Source: CAD feature listing. Evaluate the final solid. Frame: model axes, mm. Face numbers are marked on the shaded views. A direction names the side the tool comes from. Round coordinates to 2 decimals unless told otherwise and drop trailing zeros. Order: outer loops, then holes, each group sorted by start corner. A loop starts at its lowest first (then second) coordinate and runs counter-clockwise, first axis right, second up. Notation, with made-up numbers: (17.25, 18.25) -> (24.25, 18.25) arc R24 ccw to (24.25, 53.25) -> close; hole circle Ø11 at (64.5, -19). An arc over 180 degrees is marked (long way). Use a Markdown table: item, result. Add a question column.
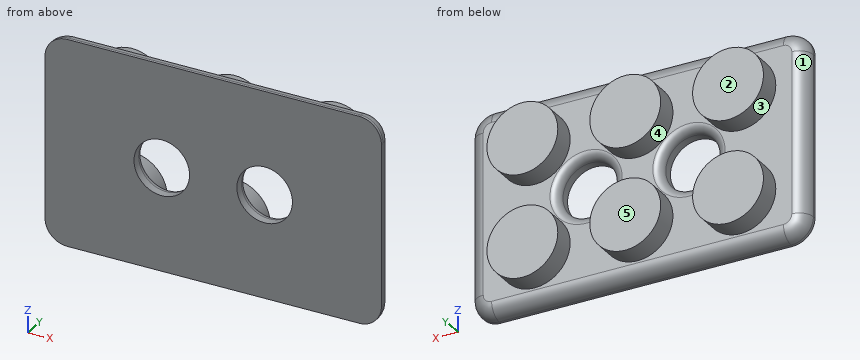
Autodesk Inventor part; units mm, degrees
ref_plane "YZ Plane" through (0, 0, 0) normal (1, 0, 0) x (0, 1, 0)
ref_plane "XZ Plane" through (0, 0, 0) normal (0, 1, 0) x (-1, 0, 0)
ref_plane "XY Plane" through (0, 0, 0) normal (0, 0, 1) x (1, 0, 0)
sketch "Sketch1" plane through (0, 0, 0) normal (0, 1, 0) x (-1, 0, 0)
  line L0 (25.9, 0) -> (-25.9, 0)
  line L1 (0, -25.9) -> (0, 25.9)
  circle A0 centre (0, 0) radius 18.5 construction
  circle A1 centre (0, 0) radius 13 construction
  dimension "d0" = 37
  dimension "d1" = 26
sketch "Sketch2" plane through (0, 0, 0) normal (0, 1, 0) x (-1, 0, 0)
  line L0 (84.7, 0) -> (-84.7, 0)
  line L1 (0, -33.3) -> (0, 70.3)
  line L2 (-60.5, 55.5) -> (-60.5, -18.5)
  line L3 (-60.5, -18.5) -> (60.5, -18.5)
  line L4 (60.5, -18.5) -> (60.5, 55.5)
  line L5 (-60.5, 55.5) -> (60.5, 55.5)
  circle A0 centre (0, 37) radius 18.5 construction
  point P0 (0, 0)
  dimension "d3" = 121
  dimension "d29" = 18.5
  dimension "d30" = 55.5
  dimension "d99" = 37
  dimension "d100" = 37
extrude "Extrusion1" add sketch "Sketch2" along normal blind 6
sketch "Sketch6" plane through (0, 0, 0) normal (0, 1, 0) x (-1, 0, 0)
  line L0 (60.5, -18.5) -> (-60.5, -18.5)
  line L1 (60.5, 55.5) -> (60.5, -18.5)
  line L2 (-60.5, -18.5) -> (60.5, -18.5)
  line L3 (60.5, -18.5) -> (60.5, 55.5)
  line L4 (-60.5, 55.5) -> (-60.5, -18.5)
  line L5 (84.7, 0) -> (-84.7, 0)
  line L6 (0, -36.3) -> (0, 70.8)
  arc A0 (-16, 0) -> (16, 0) centre (0, 0) ccw
  line L7 (16, 0) -> (16, 55.5)
  line L8 (60.5, 55.5) -> (-60.5, 55.5)
  line L9 (16, 55.5) -> (60.5, 55.5)
  line L10 (-16, 0) -> (-16, 55.5)
  line L11 (-16, 55.5) -> (-60.5, 55.5)
  point P0 (-17.3617, -21)
  dimension "d18" = 32
extrude "Extrusion5" [suppressed]
sketch "Sketch4" plane through (0, 0, 0) normal (0, 0, 1) x (1, 0, 0)
  line L0 (-18.5, 0) -> (18.5, 0)
  line L1 (18.5, 0) -> (18.5, -2)
  line L2 (18.5, -2) -> (-18.5, -2)
  line L3 (-18.5, -2) -> (-18.5, 0)
  line L4 (-25.9, 0) -> (25.9, 0)
  line L5 (0, -2.4) -> (0, 0.4)
  point P0 (0, 0)
  dimension "d10" = 37
  dimension "d11" = 2
extrude "Extrusion6" [suppressed]
sketch "Sketch5" plane through (0, 0, 0) normal (0, 1, 0) x (-1, 0, 0)
  circle A0 centre (0, 0) radius 18.5 construction
  circle A1 centre (0, 0) radius 18.5 construction
  line L0 (25.9, 0) -> (-25.9, 0)
  line L1 (0, -28.9) -> (0, 26.4)
  line L2 (-18.5, -21) -> (18.5, -21)
  line L3 (18.5, -21) -> (18.5, -18.5)
  line L4 (18.5, -18.5) -> (-18.5, -18.5)
  line L5 (-18.5, -18.5) -> (-18.5, -21)
  dimension "d25" = 37
  dimension "d26" = 21
extrude "Extrusion7" [suppressed]
sketch "Sketch7" plane through (0, 0, 0) normal (0, 0, 1) x (1, 0, 0)
  line L0 (-18.5, 0) -> (18.5, 0)
  line L1 (18.5, 0) -> (18.5, -2)
  line L2 (18.5, -2) -> (-18.5, -2)
  line L3 (-18.5, -2) -> (-18.5, 0)
  line L4 (60.5, 0) -> (-60.5, 0)
  line L5 (-84.7, 0) -> (84.7, 0)
  line L6 (0, -2.4) -> (0, 0.4)
  point P0 (-16, 0)
  point P1 (16, 0)
  dimension "d53" = 2
  dimension "d54" = 18.5
extrude "Extrusion8" [suppressed]
sketch "Sketch8" plane through (0, 0, 0) normal (0, 1, 0) x (-1, 0, 0)
  circle A0 centre (0, 0) radius 12.75
  dimension "d34" = 25.5
extrude "Extrusion9" add sketch "Sketch8" along normal blind 14
pattern_linear "Rectangular Pattern1" count 2 spacing 37 along (0, 0, 1) count 3 spacing 37 along (1, 0, 0) of "Extrusion9" second direction both ways yes
sketch "Sketch9" plane through (0, 6, 0) normal (0, 1, 0) x (1, 0, 0)
  circle A0 centre (0, 0) radius 13
  circle A1 centre (0, 0) radius 15
  dimension "d40" = 26
  dimension "d41" = 30
extrude "Extrusion10" [suppressed]
sketch "Sketch10" plane through (0, 5, 0) normal (0, 1, 0) x (1, 0, 0)
  arc A0 (16, 0) -> (-16, 0) centre (0, 0) ccw
  line L0 (1.5, -18) -> (-1.5, -18)
  line L1 (-29.4, 0) -> (29.4, 0)
  line L2 (0, 36.3) -> (0, -70.8)
  line L3 (1.5, -12) -> (-1.5, -12)
  line L4 (1.5, -12) -> (1.5, -18)
  line L5 (-1.5, -18) -> (-1.5, -12)
  dimension "d48" = 3
  dimension "d49" = 12
  dimension "d50" = 6
extrude "Extrusion11" [suppressed]
fillet "Fillet1" [suppressed]
sketch "Sketch11" plane through (0, 0, 0) normal (0, 1, 0) x (-1, 0, 0)
  line L0 (-60.5, -21) -> (60.5, -21)
  line L1 (60.5, -21) -> (60.5, -47)
  line L2 (60.5, -47) -> (-60.5, -47)
  line L3 (-60.5, -47) -> (-60.5, -21)
  line L4 (84.7, 0) -> (-84.7, 0)
  line L5 (0, -60.1) -> (0, 31.6)
  point P0 (0, 0)
  dimension "d57" = 26
  dimension "d58" = 21
  dimension "d59" = 121
extrude "Extrusion12" [suppressed]
sketch "Sketch12" plane through (0, 0, 0) normal (1, 0, 0) x (0, 1, 0)
  line L0 (6, 55.5) -> (6, -18.5)
  arc A0 (6, -16.5081) -> (5.7334, -47) centre (34, -32) ccw
  line L1 (-6.8, 0) -> (40.8, 0)
  line L2 (0, -67.5) -> (0, 76)
  line L3 (6, -16.5081) -> (6, -47)
  line L4 (6, -47) -> (5.7334, -47)
  line L5 (0, -47) -> (6, -47)
  point P0 (0, 0)
  point P1 (6, 48)
  dimension "d62" = 32
  dimension "d63" = 32
  dimension "d64" = 34
extrude "Extrusion13" [suppressed]
fillet "Fillet3" [suppressed]
sketch "Sketch13" plane through (0, 0, 0) normal (0, 1, 0) x (-1, 0, 0)
  line L0 (84.7, 0) -> (-84.7, 0)
  line L1 (0, -67.5) -> (0, 76)
  line L2 (60.5, 55.5) -> (60.5, -18.5)
  arc A0 (13.0815, 23.9185) -> (13.0815, 13.0815) centre (18.5, 18.5) ccw
  line L3 (-60.5, 55.5) -> (-60.5, -18.5)
  arc A1 (-13.0815, 13.0815) -> (-13.0815, 23.9185) centre (-18.5, 18.5) ccw
  line L4 (18.5, 37) -> (18.5, 0)
  line L5 (-18.5, 0) -> (-18.5, 37)
  line L6 (18.5, 37) -> (18.5, 55.5)
  line L7 (-60.5, 55.5) -> (60.5, 55.5)
  line L8 (-18.5, 55.5) -> (-18.5, 37)
  arc A2 (-9.2871, 53) -> (-13.0815, 23.9185) centre (0, 37) ccw
  arc A3 (13.0815, 23.9185) -> (9.2871, 53) centre (0, 37) ccw
  arc A4 (-13.0815, 13.0815) -> (-18.5, 0) centre (0, 0) ccw
  arc A5 (18.5, 0) -> (13.0815, 13.0815) centre (0, 0) ccw
  point P0 (60.5, -39.254)
  point P1 (-55.5, 48)
  point P2 (-60.5, -16.5081)
  point P3 (-60.5, -47)
  point P4 (60.5, -18.5)
  point P5 (-60.5, -18.5)
  dimension "d68" = 37
  dimension "d71" = 18.5
  dimension "d72" = 18.5
  dimension "d73" = 7.663
  dimension "d74" = 7.663
  dimension "d75" = 18.5
  dimension "d76" = 18.5
  dimension "d77" = 18.5
  dimension "d78" = 18.5
extrude "Extrusion14" [suppressed]
sketch "Sketch14" plane through (0, 0, 0) normal (0, 1, 0) x (-1, 0, 0)
  circle A0 centre (18.5, 18.5) radius 10
  line L0 (39.9, 0) -> (-39.9, 0)
  line L1 (0, -27.9) -> (0, 37.9)
  circle A1 centre (-18.5, 18.5) radius 10
  point P0 (0, 0)
  dimension "d84" = 18.5
  dimension "d85" = 18.5
  dimension "d86" = 20
  dimension "d89" = 37
extrude "Extrusion15" cut sketch "Sketch14" along normal through all
fillet "Fillet4" radius 3 2 edges at (-8.5, 6, 18.5) (28.5, 6, 18.5)
fillet "Fillet5" radius 8 4 edges at (-60.5, 3, 55.5) (60.5, 3, 55.5) (-60.5, 3, -18.5) (60.5, 3, -18.5)
fillet "Fillet6" radius 5 5 edges at (58.1569, 6, 53.1569) (60.5, 6, 18.5) (-58.1569, 6, 53.1569) (-60.5, 6, 18.5) (0, 6, 55.5)
equation "\"d85\" = d84"
properties part number "NespressoSpeedfiller-6X-tamper"
1) Section B-B on z = 18.5. Output: boundary loops of the cut face in (x, y).
2) Section D-D on z = 0. Output: boundary loops of the cut face in (x, y), then the cut area to 3 significant figures.
3) First-contact query: pin 1 Ø1.5 at (x, y) = (-2, 7) entering from +Z; pin 2 Ø1 at (x, y) = (3.5, 7.5) entering from -Z; pin 3 Ø3 at (x, y) = (39.5, 8) entering from -Z; pin 4 Ø8 at (x, y) = (34, 2.5) entering from -Z. Flat tips, straight axial feed; report the tip coordinate or a pass-through.
4) Section A-A on x = -18.5. Output: boundary loops of the cut face in (y, z), then the cut area to 3 significant figures.
5) Section C-C on y = 9. Output: boundary loops of the cut face in (x, z), then the cut area to 3 significant figures.
6) Line query: probe 1 along X at (y, z) = (0.9, 18.5); probe 2 along Z at (x, y) = (18.5, 0.9); probe 3 along X at (y, z) = (4.5, 15.5). Output: solid intervals per line, ascending. Write a range as from..to.
7) Draft query along X for the marked faces 1, 2 and 3. Return one class per face: pulls with the +X half, pulls with the -X half, needs draft (parallel to the pull), parting line crosses it, or undercut.
8) Reachability of the marked faces 4 and 5 from +Z, -Z, +X, -X, +Y, -Y: full face, straight path, thin tool, end or side. Return the list, or none.
Conclusion:
| question | item | result |
|---|---|---|
| 1 | outline | (-60.5, 0) -> (-28.5, 0) -> (-28.5, 3) arc R3 ccw to (-31.5, 6) -> (-55.5, 6) arc R5 ccw to (-60.5, 1) -> close; (-8.5, 0) -> (8.5, 0) -> (8.5, 3) arc R3 ccw to (5.5, 6) -> (-5.5, 6) arc R3 ccw to (-8.5, 3) -> close; (28.5, 0) -> (60.5, 0) -> (60.5, 1) arc R5 ccw to (55.5, 6) -> (31.5, 6) arc R3 ccw to (28.5, 3) -> close |
| 2 | outline | (-60.5, 0) -> (60.5, 0) -> (60.5, 1) arc R5 ccw to (55.5, 6) -> (49.75, 6) -> (49.75, 14) -> (24.25, 14) -> (24.25, 6) -> (12.75, 6) -> (12.75, 14) -> (-12.75, 14) -> (-12.75, 6) -> (-24.25, 6) -> (-24.25, 14) -> (-49.75, 14) -> (-49.75, 6) -> (-55.5, 6) arc R5 ccw to (-60.5, 1) -> close |
| 2 | area | 1,330 mm^2 |
| 3 | pin 1 | stops at z = 49.69 |
| 3 | pin 2 | stops at z = -12.39 |
| 3 | pin 3 | stops at z = -12.71 |
| 3 | pin 4 | stops at z = -18.5 |
| 4 | outline | (0, -18.5) -> (1, -18.5) arc R5 ccw to (6, -13.5) -> (6, 5.5) arc R3 ccw to (3, 8.5) -> (0, 8.5) -> close; (0, 28.5) -> (3, 28.5) arc R3 ccw to (6, 31.5) -> (6, 50.5) arc R5 ccw to (1, 55.5) -> (0, 55.5) -> close |
| 4 | area | 309 mm^2 |
| 5 | outline | circle Ø25.5 at (-37, 0); circle Ø25.5 at (-37, 37); circle Ø25.5 at (0, 0); circle Ø25.5 at (0, 37); circle Ø25.5 at (37, 0); circle Ø25.5 at (37, 37) |
| 5 | area | 3,060 mm^2 |
| 6 | probe 1 | x = -60.5..-28.5, -8.5..8.5, 28.5..60.5 |
| 6 | probe 2 | z = -18.5..8.5, 28.5..55.5 |
| 6 | probe 3 | x = -59.07..-28.46, -8.54..8.54, 28.46..59.07 |
| 7 | face 1 | pulls with the -X half |
| 7 | face 2 | needs draft |
| 7 | face 3 | undercut |
| 8 | face 4 | +Y |
| 8 | face 5 | +Z, -Z, +X, -X, +Y |
